The listing builds one solid part. Answer for the finished solid, in the listing's coordinates (mm). A direction names the side the tool comes from. Give positions to 0.01 mm unless a question says otherwise; leave off trailing zeros. Loops run counter-clockwise (first coordinate to the right, second up) from the corner with the lowest first, then second, coordinate; pieces in that order, holes last. Notation, with made-up numbers: M -6.75,74 L 46.25,74 A24 ccw 46.25,96 Z; hole C 50,-10.5 d2. An arc over 180 degrees is marked long. One line per item, written item: value. Start each with the question number.
Q1. A cutting plane is placed at A-A, the plane x = 4. Determine the outline of the cut face in (y, z) (3 decimals), and give its area (3 significant figures).
Q2. For faces 5 (the cylindrical face through (-12.52, -3.1, 0.69)), 6 (the flat face through (25.4, 3, -3)), 7 (the cylindrical face through (23.22, -1.38, 6.2)), determine the directions among +Z, -Z, +X, -X, +Y, -Y from which every point of the face is accessible in a straight line to the end or side of a thin tool.
Q3. A cutting plane is placed at B-B, the plane x = -21.5. Determine the outline of the cut face in (y, z) (3 decimals), and give its area (3 significant figures).
Q4. Flat-ended cylindrical pins translate along their axes: pin 1 (1 mm diameter, centred on x = 16, y = -0.5, fed in from -Z); pin 2 (3 mm diameter, centred on x = -4, z = -1.5, fed in from -Y) (3 decimals); pin 3 (3 mm diameter, centred on x = 18.5, z = 5.5, fed in from -Y). Find the tip coordinate at first contact, or state that the pin passes through.
Q5. The mould has two halves that part along X. Classify faces 1 (the cylindrical face through (7.1, 6.926, -0.909)), 2 (the cylindrical face through (-12.16, 0.73, -0.21)), 3 (the flat face through (2.54, 0, 1)), 4 (the flat face through (-25.4, -1.4, 0)): +X half, -X half, draft (parallel to the pull), parting line (faces both ways), or undercut.
Q6. Consider L1, parallel to Y at x = 10.25, z = 0 (3 decimals); L2, parallel to Z at x = 1.25, y = 0 (3 decimals). Determine where each line is inside the solid, lowest interval first.
Autodesk Inventor part; units mm, degrees
ref_plane "YZ Plane" through (0, 0, 0) normal (1, 0, 0) x (0, 1, 0)
ref_plane "XZ Plane" through (0, 0, 0) normal (0, 1, 0) x (-1, 0, 0)
ref_plane "XY Plane" through (0, 0, 0) normal (0, 0, 1) x (1, 0, 0)
sketch "Sketch1" plane through (0, 0, 0) normal (1, 0, 0) x (0, 1, 0)
  circle A0 centre (0, 0) radius 3.175
  circle A1 centre (0, 0) radius 6.35
  dimension "d0" = 6.35
  dimension "d1" = 12.7
extrude "Extrusion1" add sketch "Sketch1" along normal blind 25.4
sketch "Sketch2" plane through (25.4, 0, 0) normal (1, 0, 0) x (0, 0, -1)
  circle A0 centre (0, 0) radius 3.175
  circle A1 centre (0, 0) radius 3.175
extrude "Extrusion2" add sketch "Sketch2" against normal blind 50.8
sketch "Sketch3" plane through (0, 0, 0) normal (-1, 0, 0) x (0, 0, 1)
  circle A0 centre (0, 0) radius 9.525
  dimension "d6" = 19.05
extrude "Extrusion3" add sketch "Sketch3" against normal blind 12.7
fillet "Fillet1" radius 12.7 1 edges at (12.7, -6.35, 0)
shell "Shell1" thickness 2.54 removed faces 1 at (25.4, -1.8127, -0.4771)
hole "Hole1" at (-25.4, 0.1121, -0.0708) direction (1, 0, 0) diameter 1.27 depth 25.4 tip angle 118 countersink diameter 2.54 countersink angle 82
Answer block:
1. outline: C 0,0 d19.05; hole C 0,0 d13.97
1. area: 132 mm^2
2. face 5: -X
2. face 6: +Z, -Z, +X, +Y, -Y
2. face 7: +X
3. outline: C 0,0 d6.35; hole M -0.281,-0.569 A0.635 ccw long 0.393,0.499 A0.635 ccw long Z
3. area: 30.2 mm^2
4. pin 1: z = -7.64
4. pin 2: y = -3.175
4. pin 3: y = -5.36
5. face 1: undercut
5. face 2: draft
5. face 3: undercut
5. face 4: -X half
6. L1: -9.525 to -6.985, 6.985 to 9.525
6. L2: -9.525 to -0.635, 0.635 to 9.525
